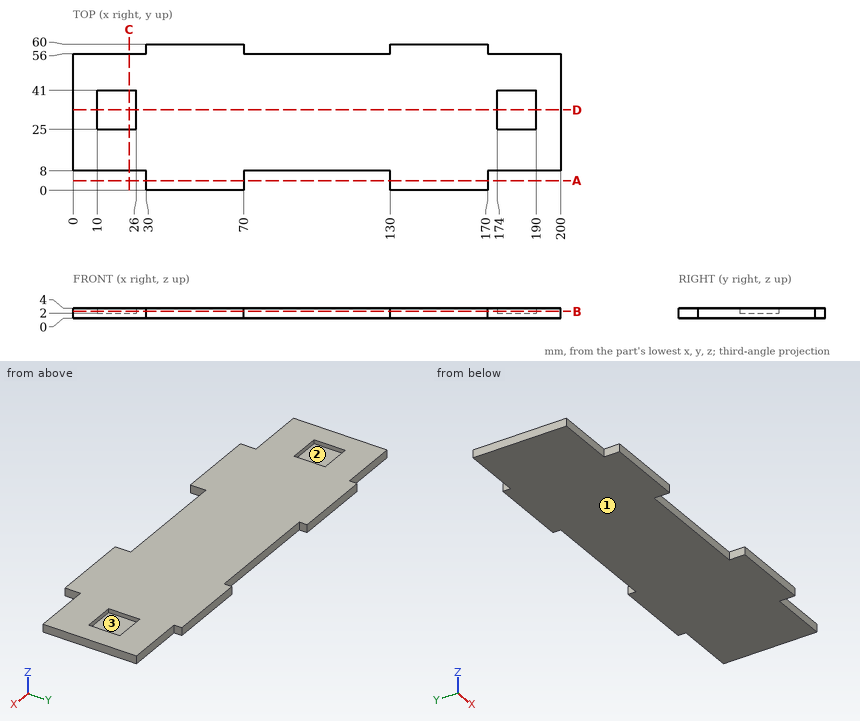
Job drawing, mm, ordinate dimensions from the low corner. One solid piece. Coordinates: 2 decimals unless noted, no trailing zeros. Loops run counter-clockwise (first coordinate to the right, second up) from the corner with the lowest first, then second, coordinate; pieces in that order, holes last. Notation, with made-up numbers: (67.25, -18) -> (91.25, -18) arc R24 cw to (91.25, 21) -> close; hole circle Ø7 at (62.5, 52.5). An arc over 180 degrees is marked (long way). One line per item, written item: value.
1. Pull direction Y, two halves, no side cores. Call the marked faces 1, 2 and 3: pulls with the +Y half, pulls with the -Y half, needs draft (parallel to the pull), parting line crosses it, or undercut.
Answers:
face 1: needs draft
face 2: undercut
face 3: undercut
2. Drill centre lines: line 1 (X direction, y = 37.5, z = 2.05); line 2 (Y direction, x = 187.5, z = 2.3); line 3 (Y direction, x = 10.5, z = 0.65). Where is each one in solid material? Low to high. Write a range as [from, to].
Answers:
line 1: x = [0, 10], [26, 174], [190, 200]
line 2: y = [8, 25], [41, 56]
line 3: y = [8, 56]
3. Flat gauge pins, fed straight in: P1, Ø2, axis at y = 3.5, z = 2.5, coming from the +X side; P2, Ø2, axis at x = 179, z = 1, coming from the +Y side; P3, Ø5, axis at x = 16, y = 33.5, coming from the +Z side. Where does each tip first touch, or does it go through?
Answers:
P1: stops at x = 170
P2: stops at y = 56
P3: stops at z = 2
4. Slice it at C-C on x = 23. Write the cut outline in (y, z).
Answers:
outline: (8, 0) -> (56, 0) -> (56, 4) -> (41, 4) -> (41, 2) -> (25, 2) -> (25, 4) -> (8, 4) -> close
5. Slice it at A-A on y = 4. Write the cut outline in (x, z), and give its area (3 significant figures).
Answers:
outline: (30, 0) -> (70, 0) -> (70, 4) -> (30, 4) -> close; (130, 0) -> (170, 0) -> (170, 4) -> (130, 4) -> close
area: 320 mm^2
6. Slice it at D-D on y = 33. Write the cut outline in (x, z), and give its area (3 significant figures).
Answers:
outline: (0, 0) -> (200, 0) -> (200, 4) -> (190, 4) -> (190, 2) -> (174, 2) -> (174, 4) -> (26, 4) -> (26, 2) -> (10, 2) -> (10, 4) -> (0, 4) -> close
area: 736 mm^2
7. Slice it at B-B on z = 2.75. Write the cut outline in (x, y).
Answers:
outline: (0, 8) -> (30, 8) -> (30, 0) -> (70, 0) -> (70, 8) -> (130, 8) -> (130, 0) -> (170, 0) -> (170, 8) -> (200, 8) -> (200, 56) -> (170, 56) -> (170, 60) -> (130, 60) -> (130, 56) -> (70, 56) -> (70, 60) -> (30, 60) -> (30, 56) -> (0, 56) -> close; hole (10, 25) -> (26, 25) -> (26, 41) -> (10, 41) -> close; hole (174, 25) -> (190, 25) -> (190, 41) -> (174, 41) -> close
